Could you check a few things on this model? Use its own coordinates, in mm. A direction names the side the tool comes from. Coordinates: 2 decimals unless noted, no trailing zeros. Order: outer loops, then holes, each group sorted by start corner. A loop starts at its lowest first (then second) coordinate and runs counter-clockwise, first axis right, second up. Notation, with made-up numbers: (-8.5, 41.5) -> (32.5, 41.5) arc R27 ccw to (32.5, 69.5) -> close; hole circle Ø4 at (36.25, 75.5). An arc over 180 degrees is marked (long way). Use a Markdown table: item, result. Add a question column.
1) If I drill on L1, parallel to Y at x = 261, z = 33; L2, parallel to X at y = -59, z = 55; L3, parallel to Y at x = 114, z = 27, over which ranges is the centre line in solid material (lowest first)? Write a range as [from, to].
2) Will these pins go through, and if not, where does the flat tip stop? pin 1 Ø10 at (x, y) = (66, -83) entering from +Z; pin 2 Ø10 at (x, y) = (152, -49) entering from -Z; pin 3 Ø6.5 at (x, y) = (278.5, -8) entering from +Z; pin 4 Ø4 at (y, z) = (-43, 22) entering from +X.
3) Which directions (+Z, -Z, +X, -X, +Y, -Y) give clear straight access to the entire face, cutting with the end or side of a thin tool? Please do faces 4 (the flat face through (170, -84, 29.21)), 5 (the cylindrical face through (283.316, -62.901, 101.234)), 6 (the flat face through (283, -118, 55.88)).
4) Thinking about a two-plate mould opening in Z: for faces 1 (the flat face through (170, -36, 29.21)), 2 (the flat face through (31.75, -63, 69)), 3 (the flat face through (6.76, -62.61, 94.89)), which applies, +Z half, -Z half, draft (parallel to the pull), parting line (faces both ways), or undercut?
5) If we section it at C-C (y = -117): Write out the boundary of the cut face in (x, z).
6) If we section it at A-A (x = 163.5): Write out the boundary of the cut face in (y, z), plus the area to 3 significant figures.
7) If we section it at B-B (z = 46): Write out the boundary of the cut face in (x, y), plus the area to 3 significant figures.
8) If we section it at D-D (z = 10.5): Write out the boundary of the cut face in (x, y), plus the area to 3 significant figures.
```python
from build123d import *

# Parameters (mm, degrees)
F1_DEPTH = 127
F3_DEPTH = 38.354
F4_R     = 12.7
F5_DEPTH = 63.5
F7_DEPTH = 272.796
F8_R     = 5.08


with BuildPart() as f1:
    # F0 (on Front) → F1 (new body)
    with BuildSketch(Plane.XZ):
        Polygon((0, 87.987836793), (0, 0), (304.8, 0), (304.8, 55.88), (266.7, 55.88), (266.7, 38.1), (31.75, 38.1), (31.75, 101.6), (13.3270969392, 101.6), align=None)
    extrude(amount=F1_DEPTH)

    # F2 (on face) → F3 (join)
    with BuildSketch(Plane.YZ.offset(304.8)):
        with BuildLine():
            Line((-83.2950948956, 91.4038064892), (-110.8501477266, 55.88))
            Line((-110.8501477266, 55.88), (-15.6001477266, 55.88))
            Line((-15.6001477266, 55.88), (-43.1552005575, 91.4038064892))
            ThreePointArc((-43.1552005575, 91.4038064892), (-63.2251477266, 101.2359800311), (-83.2950948956, 91.4038064892))
        make_face()
    extrude(amount=-F3_DEPTH)

    # F4 (on face) → F5 (cut, symmetric)
    with BuildSketch(Plane.YZ.offset(304.8)):
        with Locations((-63.2251477266, 75.8359800311)):
            Circle(F4_R)
    extrude(amount=F5_DEPTH, both=True, mode=Mode.SUBTRACT)

    # F6 (on face) → F7 (cut)
    with BuildSketch(Plane.YZ.offset(304.8)):
        Polygon((-75.8447764756, 16.51), (-75.8447764756, 0), (-44.662312481, 0), (-44.662312481, 16.51), (-28.5035444783, 16.51), (-28.5035444783, 29.21), (-44.662312481, 29.21), (-44.662312481, 38.1537896351), (-75.8601041585, 38.1), (-75.8447764756, 29.21), (-92.0035444783, 29.21), (-92.0035444783, 16.51), align=None)
    extrude(amount=-F7_DEPTH, mode=Mode.SUBTRACT)

    # F8
    f8_edges = [f1.edges().sort_by_distance(p)[0] for p in [
        (304.8, -97.072621, 73.641903),
        (304.8, -7.800074, 55.88),
        (304.8, -118.925074, 55.88),
        (285.75, -127, 55.88),
        (285.623, -83.295095, 91.403806),
        (285.623, -43.155201, 91.403806),
        (304.8, -29.377674, 73.641903),
        (304.8, -63.225148, 101.23598),
        (285.75, -15.600148, 55.88),
        (285.75, -110.850148, 55.88),
    ]]
    fillet(f8_edges, radius=F8_R)


solid = f1.part
```
Answer sheet:
| question | item | result |
|---|---|---|
| 1 | L1 | [-127, -75.85], [-44.66, 0] |
| 1 | L2 | [0, 31.75], [266.7, 304.8] |
| 1 | L3 | [-127, -92], [-28.5, 0] |
| 2 | pin 1 | z = 38.1 |
| 2 | pin 2 | z = 0 |
| 2 | pin 3 | z = 55.88 |
| 2 | pin 4 | x = 32 |
| 3 | face 4 | +X |
| 3 | face 5 | +Z, +X |
| 3 | face 6 | +Z, +X, -Y |
| 4 | face 1 | undercut |
| 4 | face 2 | draft |
| 4 | face 3 | +Z half |
| 5 | outline | (0, 0) -> (304.8, 0) -> (304.8, 50.8) arc R5.08 ccw to (299.72, 55.88) -> (266.7, 55.88) -> (266.7, 38.1) -> (31.75, 38.1) -> (31.75, 101.6) -> (13.33, 101.6) -> (0, 87.99) -> close |
| 6 | outline | (-127, 0) -> (-75.84, 0) -> (-75.84, 16.51) -> (-92, 16.51) -> (-92, 29.21) -> (-75.84, 29.21) -> (-75.86, 38.1) -> (-127, 38.1) -> close; (-44.66, 0) -> (0, 0) -> (0, 38.1) -> (-44.66, 38.1) -> (-44.66, 29.21) -> (-28.5, 29.21) -> (-28.5, 16.51) -> (-44.66, 16.51) -> close |
| 6 | area | 3,240 mm2 |
| 7 | outline | (0, -127) -> (31.75, -127) -> (31.75, 0) -> (0, 0) -> close; (266.7, -127) -> (304.8, -127) -> (304.8, 0) -> (266.7, 0) -> close |
| 7 | area | 8,870 mm2 |
| 8 | outline | (0, -127) -> (304.8, -127) -> (304.8, -75.84) -> (32, -75.84) -> (32, -44.66) -> (304.8, -44.66) -> (304.8, 0) -> (0, 0) -> close |
| 8 | area | 30,200 mm2 |
